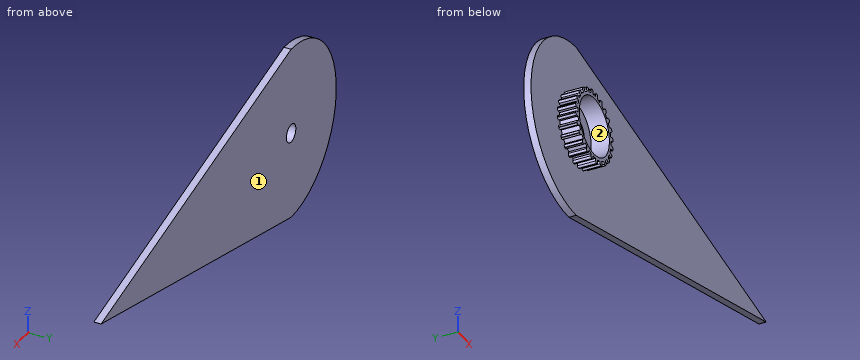
from build123d import *

# Parameters (mm, degrees)
BOSS_EXTRUDE1_DEPTH      = 2
SKETCH2_R                = 10
SKETCH2_R_2              = 8
BOSS_EXTRUDE2_DEPTH      = 5
SKETCH4_R                = 3.25
BOSS_EXTRUDE3_DEPTH      = 0.5
SKETCH5_R                = 2.5
CUT_EXTRUDE2_DEPTH       = 2.5
CUT_EXTRUDE3_DEPTH       = 5
FILLET1_R                = 0.5
CIRPATTERN5_COUNT        = 24
FILLET1_OF_CIRPATTERN5_R = 0.5


with BuildPart() as part:
    # Sketch1 → Boss-Extrude1 (new body)
    with BuildSketch(Plane(origin=(0, 0, 0), x_dir=(1, 0, 0), z_dir=(0, 1, 0))):
        with BuildLine():
            Line((0, 24), (101, 0))
            Line((101, 0), (0, -24))
            ThreePointArc((0, -24), (-24, 0), (0, 24))
        make_face()
    extrude(amount=BOSS_EXTRUDE1_DEPTH)

    # Sketch2 → Boss-Extrude2 (add)
    with BuildSketch(Plane.XZ):
        with Locations(Location((0, 0, 0), (0, 0, 270))):
            Circle(SKETCH2_R)
        with Locations(Location((0, 0, 0), (0, 0, 270))):
            Circle(SKETCH2_R_2, mode=Mode.SUBTRACT)
    extrude(amount=BOSS_EXTRUDE2_DEPTH)

    # Sketch4 → Boss-Extrude3 (add)
    with BuildSketch(Plane(origin=(0, 0, 0), x_dir=(-1, 0, 0), z_dir=(0, -1, 0))):
        with Locations(Location((0, 0, 0), (0, 0, 270))):
            Circle(SKETCH4_R)
    extrude(amount=BOSS_EXTRUDE3_DEPTH)

    # Sketch5 → Cut-Extrude2 (cut)
    with BuildSketch(Plane.XZ.offset(0.5)):
        with Locations(Location((0, 0, 0), (0, 0, 270))):
            Circle(SKETCH5_R)
    extrude(amount=-CUT_EXTRUDE2_DEPTH, mode=Mode.SUBTRACT)

    # Sketch6 → Cut-Extrude3 (cut)
    with BuildSketch(Plane.XZ.offset(5)):
        Polygon((-1, 11.817203407), (1, 11.817203407), (0.586202372, 8.817203407), (-0.586202372, 8.817203407), align=None)
    cut_extrude3 = extrude(amount=-CUT_EXTRUDE3_DEPTH, mode=Mode.SUBTRACT)

    # Fillet1
    fillet1_edges = [part.edges().sort_by_distance(p)[0] for p in [
        (0.745510128, -2.5, 9.972172013),
        (-0.745510128, -2.5, 9.972172013),
    ]]
    fillet(fillet1_edges, radius=FILLET1_R)

    # CirPattern5: Cut-Extrude3 ×24 about axis
    cirpattern5_axis = Axis((0, 0, 0), (0, 1, 0))
    for i in range(1, CIRPATTERN5_COUNT):
        add(cut_extrude3.rotate(cirpattern5_axis, i * 360 / CIRPATTERN5_COUNT), mode=Mode.SUBTRACT)

    # Fillet1 of CirPattern5
    fillet1_of_cirpattern5_edges = [part.edges().sort_by_distance(p)[0] for p in [
        (3.301095525, -2.5, 9.439426272),
        (1.860880551, -2.5, 9.825330711),
        (5.631716716, -2.5, 8.26339923),
        (4.340455296, -2.5, 9.008909358),
        (7.57854572, -2.5, 6.524235186),
        (6.524235186, -2.5, 7.57854572),
        (9.008909358, -2.5, 4.340455296),
        (8.26339923, -2.5, 5.631716716),
        (9.825330711, -2.5, 1.860880551),
        (9.439426272, -2.5, 3.301095525),
        (9.972172013, -2.5, -0.745510128),
        (9.972172013, -2.5, 0.745510128),
        (9.439426272, -2.5, -3.301095525),
        (9.825330711, -2.5, -1.860880551),
        (8.26339923, -2.5, -5.631716716),
        (9.008909358, -2.5, -4.340455296),
        (6.524235186, -2.5, -7.57854572),
        (7.57854572, -2.5, -6.524235186),
        (4.340455296, -2.5, -9.008909358),
        (5.631716716, -2.5, -8.26339923),
        (1.860880551, -2.5, -9.825330711),
        (3.301095525, -2.5, -9.439426272),
        (-0.745510128, -2.5, -9.972172013),
        (0.745510128, -2.5, -9.972172013),
        (-3.301095525, -2.5, -9.439426272),
        (-1.860880551, -2.5, -9.825330711),
        (-5.631716716, -2.5, -8.26339923),
        (-4.340455296, -2.5, -9.008909358),
        (-7.57854572, -2.5, -6.524235186),
        (-6.524235186, -2.5, -7.57854572),
        (-9.008909358, -2.5, -4.340455296),
        (-8.26339923, -2.5, -5.631716716),
        (-9.825330711, -2.5, -1.860880551),
        (-9.439426272, -2.5, -3.301095525),
        (-9.972172013, -2.5, 0.745510128),
        (-9.972172013, -2.5, -0.745510128),
        (-9.439426272, -2.5, 3.301095525),
        (-9.825330711, -2.5, 1.860880551),
        (-8.26339923, -2.5, 5.631716716),
        (-9.008909358, -2.5, 4.340455296),
        (-6.524235186, -2.5, 7.57854572),
        (-7.57854572, -2.5, 6.524235186),
        (-4.340455296, -2.5, 9.008909358),
        (-5.631716716, -2.5, 8.26339923),
        (-1.860880551, -2.5, 9.825330711),
        (-3.301095525, -2.5, 9.439426272),
    ]]
    fillet(fillet1_of_cirpattern5_edges, radius=FILLET1_OF_CIRPATTERN5_R)


solid = part.part
The listing builds one solid part. Answer for the finished solid, in the listing's coordinates (mm). Face numbers are marked on the shaded views. Give positions to 0.01 mm unless a question says otherwise; leave off trailing zeros. Write each loop counter-clockwise with the first axis right and the second up, starting at its lowest first coordinate (ties: lowest second). Pieces come first, ordered by that corner, then holes.
Item 1: Find the intervals of material crossed by line 1 along X through (y, z) = (-1.2, 0); line 2 along Y through (x, z) = (71, 1); line 3 along Z through (x, y) = (-5, -1) (3 decimals), in increasing order.
Item 2: Flat-ended cylindrical pins translate along their axes: P1, Ø2, axis at y = 0, z = -18.5, coming from the -X side; P2, Ø6, axis at x = 0, z = 0, coming from the -Y side; P3, Ø24, axis at x = 25, z = 11, coming from the -Y side. Find the tip coordinate at first contact, or state that the pin passes through.
Item 3: Section B-B, the plane z = 15 is taken. Write down the section's boundary in (x, y) (3 decimals), plus the area to 3 significant figures.
Item 4: Determine the mould class of the marked faces 1 and 2 for opening direction X: released by +X, released by -X, zero draft, split by the parting line, or undercut.
Item 5: Section A-A, the plane x = 87 is taken. Write down the section's boundary in (y, z).
Completed:
1. line 1: x = -8.82 to -8, 8 to 8.82
1. line 2: y = 0 to 2
1. line 3: z = -7.451 to -6.245, 6.245 to 7.451
2. P1: stops at x = -16.42
2. P2: stops at y = -0.5
2. P3: stops at y = 0
3. outline: (-18.735, 0) - (37.875, 0) - (37.875, 2) - (-18.735, 2) - close
3. area: 113 mm2
4. face 1: zero draft
4. face 2: undercut
5. outline: (0, -3.33) - (2, -3.33) - (2, 3.33) - (0, 3.33) - close
